The model under review builds one solid part; all positions refer to its coordinate system, in mm. A direction names the side the tool comes from. Give positions to 0.01 mm unless a question says otherwise; leave off trailing zeros. Order: outer loops, then holes, each group sorted by start corner. A loop starts at its lowest first (then second) coordinate and runs counter-clockwise, first axis right, second up. Notation, with made-up numbers: (11, 21) -> (22, 21) arc R35 ccw to (22, 56) -> close; hole circle Ø1 at (-11, 54). An arc over 180 degrees is marked (long way). Use one line per item in the form item = value.
```python
from build123d import *

# Parameters (mm, degrees)
F0_W           = 76.2
F0_H           = 50.8
F1_DEPTH       = 6.35
F2_W           = 76.2
F2_H           = 5.08
F3_DEPTH       = 101.6
F4_R           = 6.477
F5_DEPTH       = 50.801
F4_R_2         = 1.2
F4_R_3         = 3.5
F6_DEPTH       = 5.08
F8_DEPTH       = 16.002
F9_R           = 12.446
F9_R_2         = 1.2
F9_R_3         = 3.5
F10_DEPTH      = 3.175
F12_DEPTH      = 19.177
F14_DEPTH      = 38.101
F14_DEPTH_BACK = 38.101


# Not quite as in the source:
# - a feature names something its author has since deleted; it is built from what else it names


with BuildPart() as f1:
    # F0 (on Top) → F1 (new body)
    with BuildSketch(Plane.XY):
        Rectangle(F0_W, F0_H)
        with BuildLine():
            ThreePointArc((-31.75, -8.255), (-30.2621024484, -4.6628975516), (-26.67, -3.175))
            Line((-26.67, -3.175), (-8.255, -3.175))
            ThreePointArc((-8.255, -3.175), (-4.6628975516, -4.6628975516), (-3.175, -8.255))
            Line((-3.175, -8.255), (-3.175, -13.97))
            ThreePointArc((-3.175, -13.97), (-4.6628975516, -17.5621024484), (-8.255, -19.05))
            Line((-8.255, -19.05), (-26.67, -19.05))
            ThreePointArc((-26.67, -19.05), (-30.2621024484, -17.5621024484), (-31.75, -13.97))
            Line((-31.75, -13.97), (-31.75, -8.255))
        make_face(mode=Mode.SUBTRACT)
        with BuildLine():
            ThreePointArc((8.255, -19.05), (4.6628975516, -17.5621024484), (3.175, -13.97))
            Line((3.175, -13.97), (3.175, -8.255))
            ThreePointArc((3.175, -8.255), (4.6628975516, -4.6628975516), (8.255, -3.175))
            Line((8.255, -3.175), (26.67, -3.175))
            ThreePointArc((26.67, -3.175), (30.2621024484, -4.6628975516), (31.75, -8.255))
            Line((31.75, -8.255), (31.75, -13.97))
            ThreePointArc((31.75, -13.97), (30.2621024484, -17.5621024484), (26.67, -19.05))
            Line((26.67, -19.05), (8.255, -19.05))
        make_face(mode=Mode.SUBTRACT)
        with BuildLine():
            ThreePointArc((-31.75, 13.97), (-30.2621024484, 17.5621024484), (-26.67, 19.05))
            Line((-26.67, 19.05), (-8.255, 19.05))
            ThreePointArc((-8.255, 19.05), (-4.6628975516, 17.5621024484), (-3.175, 13.97))
            Line((-3.175, 13.97), (-3.175, 8.255))
            ThreePointArc((-3.175, 8.255), (-4.6628975516, 4.6628975516), (-8.255, 3.175))
            Line((-8.255, 3.175), (-26.67, 3.175))
            ThreePointArc((-26.67, 3.175), (-30.2621024484, 4.6628975516), (-31.75, 8.255))
            Line((-31.75, 8.255), (-31.75, 13.97))
        make_face(mode=Mode.SUBTRACT)
        with BuildLine():
            Line((31.75, 13.97), (31.75, 8.255))
            ThreePointArc((31.75, 8.255), (30.2621024484, 4.6628975516), (26.67, 3.175))
            Line((26.67, 3.175), (8.255, 3.175))
            ThreePointArc((8.255, 3.175), (4.6628975516, 4.6628975516), (3.175, 8.255))
            Line((3.175, 8.255), (3.175, 13.97))
            ThreePointArc((3.175, 13.97), (4.6628975516, 17.5621024484), (8.255, 19.05))
            Line((8.255, 19.05), (26.67, 19.05))
            ThreePointArc((26.67, 19.05), (30.2621024484, 17.5621024484), (31.75, 13.97))
        make_face(mode=Mode.SUBTRACT)
    extrude(amount=F1_DEPTH)

    # F2 (on face) → F3 (join)
    with BuildSketch(Plane.XY.offset(6.35)):
        with Locations((0, 22.86)):
            Rectangle(F2_W, F2_H)
        with Locations((0, -22.86)):
            Rectangle(F2_W, F2_H)
    extrude(amount=F3_DEPTH)

    # F4 (on face) → F5 (cut, through all)
    with BuildSketch(Plane.XZ.offset(25.4)):
        with BuildLine():
            Line((28.0908644484, 41.5545914238), (38.1, 6.35))
            Line((38.1, 6.35), (38.1, 107.95))
            Line((38.1, 107.95), (-38.1, 107.95))
            Line((-38.1, 107.95), (-38.1, 6.35))
            Line((-38.1, 6.35), (-24.5981673582, 42.522585505))
            ThreePointArc((-24.5981673582, 42.522585505), (-13.2952924023, 50.7674986335), (-1.27, 43.6172596583))
            ThreePointArc((-1.27, 43.6172596583), (1.5875, 41.8262100729), (4.445, 43.6172596583))
            ThreePointArc((4.445, 43.6172596583), (16.9786511198, 50.7334125607), (28.0908644484, 41.5545914238))
        make_face()
        with Locations((-12.7, 38.081458)):
            Circle(F4_R)
    extrude(amount=-F5_DEPTH, mode=Mode.SUBTRACT)

    # F4 (on face) → F6 (cut, through all)
    with BuildSketch(Plane.XZ.offset(25.4)):
        with Locations((-3.175, 38.081458)):
            Circle(F4_R_2)
        with Locations((-22.225, 38.081458)):
            Circle(F4_R_2)
        with Locations((15.875, 38.081458)):
            Circle(F4_R_3)
    extrude(amount=-F6_DEPTH, mode=Mode.SUBTRACT)

    # F7 (on face) → F8 (join)
    with BuildSketch(Plane.XZ.offset(25.4)):
        with BuildLine():
            ThreePointArc((25.781, 38.081458), (15.875, 28.175458), (5.969, 38.081458))
            Line((5.969, 38.081458), (5.969, 45.6163156629))
            ThreePointArc((5.969, 45.6163156629), (15.875, 25.635458), (25.781, 45.6163156629))
            Line((25.781, 45.6163156629), (25.781, 38.081458))
        make_face()
    extrude(amount=F8_DEPTH)

    # F9 (on face) → F10 (join)
    with BuildSketch(Plane.XZ.offset(41.402)):
        with Locations((15.875, 38.081458)):
            Circle(F9_R)
        with Locations((6.35, 38.081458)):
            Circle(F9_R_2, mode=Mode.SUBTRACT)
        with Locations((15.875, 38.081458)):
            Circle(F9_R_3, mode=Mode.SUBTRACT)
        with Locations((25.4, 38.081458)):
            Circle(F9_R_2, mode=Mode.SUBTRACT)
    extrude(amount=F10_DEPTH)

    # F11 (on face) → F12 (join, through all)
    with BuildSketch(Plane.XZ.offset(25.4)):
        with BuildLine():
            Line((4.5542674961, 32.9100044737), (15.875, 8.128))
            Line((15.875, 8.128), (27.1957325039, 32.9100044737))
            ThreePointArc((27.1957325039, 32.9100044737), (15.875, 25.635458), (4.5542674961, 32.9100044737))
        make_face()
    extrude(amount=F12_DEPTH)

    # F13 (on Right) → F14 (cut, two sides)
    with BuildSketch(Plane.YZ) as f14_sk:
        Polygon((-25.4, 8.128), (-44.577, 30.9822586452), (-44.577, 8.128), align=None)
    extrude(amount=-F14_DEPTH, mode=Mode.SUBTRACT)
    extrude(f14_sk.sketch, amount=F14_DEPTH_BACK, mode=Mode.SUBTRACT)


solid = f1.part
```
1. Add section A-A on y = -12. Give the boundary of the cut face in (x, z) (3 decimals).
Values:
outline = (-38.1, 0) -> (-31.75, 0) -> (-31.75, 6.35) -> (-38.1, 6.35) -> close; (-3.175, 0) -> (3.175, 0) -> (3.175, 6.35) -> (-3.175, 6.35) -> close; (31.75, 0) -> (38.1, 0) -> (38.1, 6.35) -> (31.75, 6.35) -> close
2. For pin 1 Ø15 at (x, z) = (-12.7, 38.08) entering from -Y; pin 2 Ø2.5 at (y, z) = (-36, 40) entering from -X; pin 3 Ø1.5 at (x, y) = (-2, 5) entering from +Z; pin 4 Ø3 at (x, z) = (24.5, 30.5) entering from -Y, all flat-tipped, find the tip position at first contact; note any pin that passes through.
Values:
pin_1 = -25.4
pin_2 = 3.45
pin_3 = 6.35
pin_4 = -44.58
3. Tool access review of faces 3 (the face through (-17, 3.175, 3)), 4 (the face through (-1, -25.4, 19)), 5 (the face through (-1, 0, 6.35)), 6 (the face through (15.42, -22.9, 41.55)): name each direction out of +Z, -Z, +X, -X, +Y, -Y from which nothing blocks a thin tool from reaching the whole face with its end or side.
Values:
face_3 = +Z, -Z
face_4 = none
face_5 = +Z, +X, -X
face_6 = -Y
4. Add section B-B on x = -12.7. Give the boundary of the cut face in (y, z) (3 decimals).
Values:
outline = (-25.4, 0) -> (-19.05, 0) -> (-19.05, 6.35) -> (-20.32, 6.35) -> (-20.32, 31.604) -> (-25.4, 31.604) -> close; (-25.4, 44.558) -> (-20.32, 44.558) -> (-20.32, 50.781) -> (-25.4, 50.781) -> close; (-3.175, 0) -> (3.175, 0) -> (3.175, 6.35) -> (-3.175, 6.35) -> close; (19.05, 0) -> (25.4, 0) -> (25.4, 31.604) -> (20.32, 31.604) -> (20.32, 6.35) -> (19.05, 6.35) -> close; (20.32, 44.558) -> (25.4, 44.558) -> (25.4, 50.781) -> (20.32, 50.781) -> close
5. For L1, parallel to Y at x = 7.5, z = 45; L2, parallel to Y at x = -31, z = 10.5; L3, parallel to Z at x = -12.7, y = -22.6, list the stretches that pass through material, from the lowest coordinate up.
Values:
L1 = -44.58 to -41.4, -25.4 to -20.32, 20.32 to 25.4
L2 = -25.4 to -20.32, 20.32 to 25.4
L3 = 0 to 31.6, 44.56 to 50.78
6. The part is to be moulded in two halves that separate along Y. For faces 1 (the face through (-1, 20.32, 23)), 2 (the face through (25.954, -42.967, 37.017)), say which applies: +Y half, -Y half, draft (parallel to the pull), parting line (faces both ways), or undercut.
Values:
face_1 = undercut
face_2 = draft
7. Add section D-D on y = -22.5. Count the separate pieces of the cut face and the enclosed holes in it, then the cut area to 3 significant figures.
Values:
separate_pieces = 1
enclosed_holes = 4
area = 2,910 mm^2
8. Add section C-C on z = 22.5. Give the boundary of the cut face in (x, y), then the cut area to 3 significant figures.
Values:
outline = (-32.07, -25.4) -> (9.31, -25.4) -> (9.31, -37.46) -> (22.44, -37.46) -> (22.44, -25.4) -> (33.51, -25.4) -> (33.51, -20.32) -> (-32.07, -20.32) -> close; (-32.07, 20.32) -> (33.51, 20.32) -> (33.51, 25.4) -> (-32.07, 25.4) -> close
area = 825 mm^2
